Could you check a few things on this drawing? It's one solid part, dimensions in mm from its lowest x, y, z. A direction names the side the tool comes from. Coordinates: 2 decimals unless noted, no trailing zeros. Order: outer loops, then holes, each group sorted by start corner. A loop starts at its lowest first (then second) coordinate and runs counter-clockwise, first axis right, second up. Notation, with made-up numbers: M 19,-7.5 L 51,-7.5 A17 cw 51,5.5 Z; hole C 33,65.5 d4. An arc over 180 degrees is marked long. One line per question, with ' | ' between items. Start each with the question number.
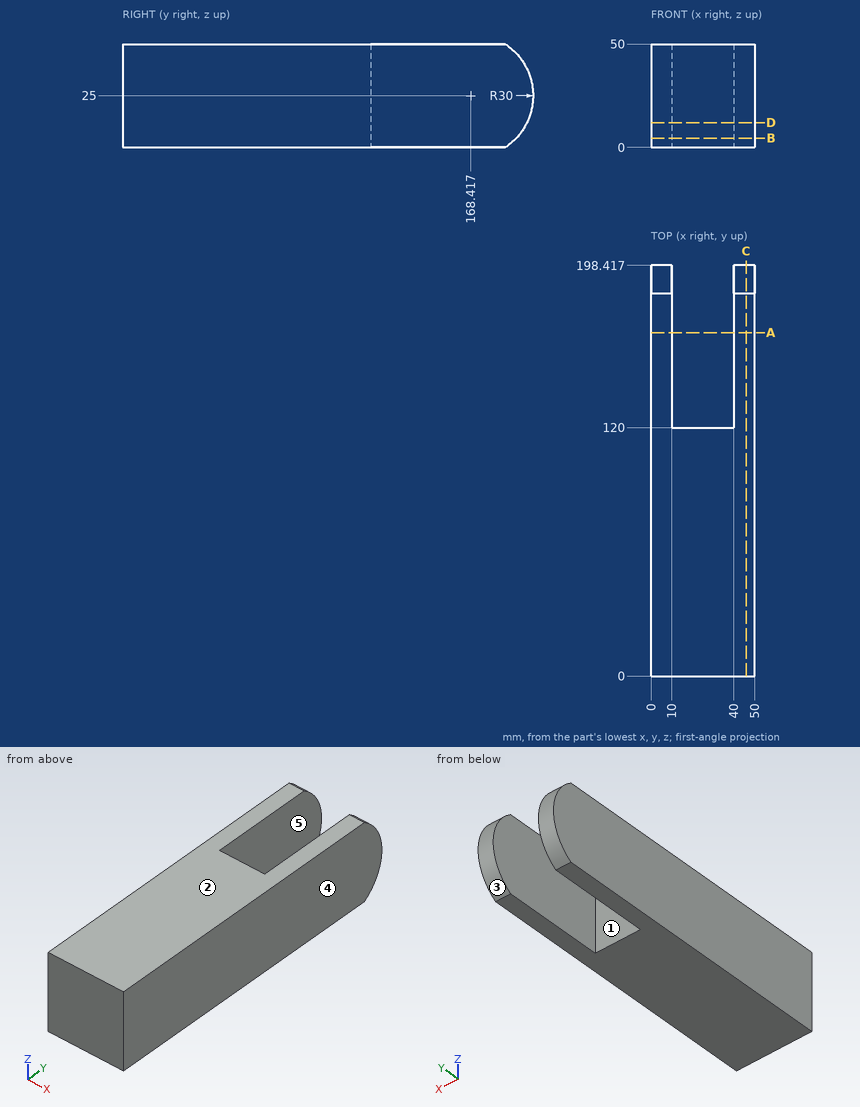
1. Will these pins go through, and if not, where does the flat tip stop? pin 1 (15 mm diameter, centred on x = 23.5, z = 35.5, fed in from +Y); pin 2 (3 mm diameter, centred on x = 21, z = 12.5, fed in from -Y).
2. Imagine slicing it at A-A (y = 166). List the corners of the cut face in (x, z) for me, then the cut area to 3 significant figures.
3. Imagine slicing it at B-B (z = 4.5). List the corners of the cut face in (x, y) for me.
4. Imagine slicing it at D-D (z = 12). List the corners of the cut face in (x, y) for me, then the cut area to 3 significant figures.
5. We'd pull the mould along X, two halves only. Please class the marked faces 3, 4 and 5: released by +X, released by -X, zero draft, split by the parting line, or undercut.
6. Imagine slicing it at C-C (x = 46). List the corners of the cut face in (y, z) for me.
7. Which directions (+Z, -Z, +X, -X, +Y, -Y) give clear straight access to the entire face, cutting with the end or side of a thin tool? Please do the marked faces 1 and 2.
8. I need wall thicknesses on line 1 (X direction, y = 190.5, z = 24); line 2 (Y direction, x = 30, z = 19); line 3 (Y direction, x = 7, z = 31). Which ranges of each line are inside material? Lowest first, please.
Entries:
1) pin 1: y = 120 | pin 2: y = 0
2) outline: M 0,0 L 10,0 L 10,50 L 0,50 Z; M 40,0 L 50,0 L 50,50 L 40,50 Z | area: 1,000 mm²
3) outline: M 0,0 L 50,0 L 50,190.32 L 40,190.32 L 40,120 L 10,120 L 10,190.32 L 0,190.32 Z
4) outline: M 0,0 L 50,0 L 50,195.45 L 40,195.45 L 40,120 L 10,120 L 10,195.45 L 0,195.45 Z | area: 7,510 mm²
5) face 3: zero draft | face 4: released by +X | face 5: undercut
6) outline: M 0,0 L 185,0 A30 ccw 185,50 L 0,50 Z
7) face 1: +Z, -Z, +Y | face 2: +Z, +X, -X, +Y, -Y
8) line 1: 0 to 10, 40 to 50 | line 2: 0 to 120 | line 3: 0 to 197.81
